Can you work these out from the model? Positions are in its coordinate system, mm. Face numbers are marked on the shaded views. Give positions to 0.01 mm unless a question says otherwise; leave off trailing zeros. Write each loop counter-clockwise with the first axis right and the second up, starting at its lowest first coordinate (ties: lowest second). Pieces come first, ordered by that corner, then holes.
Autodesk Inventor part; units mm, degrees
ref_plane "YZ Plane" through (0, 0, 0) normal (1, 0, 0) x (0, 1, 0)
ref_plane "XZ Plane" through (0, 0, 0) normal (0, 1, 0) x (-1, 0, 0)
ref_plane "XY Plane" through (0, 0, 0) normal (0, 0, 1) x (1, 0, 0)
sketch "Sketch1" plane through (-26.51, 3.1066, 0) normal (0, 0, 1) x (1, 0, 0)
  circle A0 centre (0, 0) radius 7.62 construction
  circle A1 centre (0, 0) radius 9.75
  circle A2 centre (33.02, 0) radius 25.4 construction
  line L0 (0, 0) -> (7.62, 0)
  line L1 (0, 0) -> (7.62, 0) construction
  circle A3 centre (33.02, 0) radius 9.5
  line L2 (0, -30) -> (33.02, -30)
  line L3 (33.02, 30) -> (0, 30)
  arc A4 (33.02, -30) -> (63.02, 0) centre (33.02, 0) ccw
  arc A5 (0, 30) -> (0, -30) centre (0, 0) ccw
  circle A6 centre (0, 0) radius 25.4 construction
  line L4 (0, 25.4) -> (0, 0) construction
  line L5 (0, 25.4) -> (25.4, 25.4) construction
  circle A7 centre (0, 25.4) radius 2.2
  circle A8 centre (-21.997, 12.7) radius 2.2
  circle A9 centre (-21.997, -12.7) radius 2.2
  circle A10 centre (0, -25.4) radius 2.2
  circle A11 centre (21.997, -12.7) radius 2.2
  circle A12 centre (21.997, 12.7) radius 2.2
  line L6 (63.02, 0) -> (63.02, 30)
  line L7 (63.02, 30) -> (33.02, 30)
  circle A13 centre (58.02, 25) radius 2.2
  circle A14 centre (73.02, 0) radius 2.75
  circle A15 centre (73.02, 0) radius 10
  line L8 (81.02, 6) -> (63.02, 30)
  line L9 (78.02, -8.6603) -> (48.02, -25.9808)
  dimension "d13" = 50.8
  dimension "d21" = 15.24
  dimension "d20" = 19.5
  dimension "d18" = 50.8
  dimension "d17" = 7.62
  dimension "d25" = 0
  dimension "d19" = 33.02
  dimension "d16" = 19
  dimension "d14" = 30
  dimension "d15" = 60
  dimension "d26" = 25.4
  dimension "d27" = 90
  dimension "d12" = 4.4
  dimension "d2" = 360
  dimension "d11" = 30
  dimension "d9" = 30
  dimension "d10" = 90
  dimension "d6" = 4.4
  dimension "d8" = 5
  dimension "d7" = 5
  dimension "d4" = 5.5
  dimension "d5" = 10
  dimension "d3" = 20
extrude "Extrusion1" add sketch "Sketch1" along normal blind 7 contours A5 L3 L7 L6 A4 L2 | A4 A15 L9 | L6 L8 A15 | A15 | A11 | A12
fillet "Fillet1" radius 10 1 edges at (36.51, 33.1066, 3.5)
sketch "Sketch2" plane through (-26.51, 3.1066, 7) normal (0, 0, 1) x (1, 0, 0)
  circle A0 centre (0, 25.4) radius 2.2
  circle A1 centre (0, -25.4) radius 2.2
  circle A2 centre (58.02, 25) radius 2.2
  point P0 (26.51, -3.1066)
hole "Hole1" at (-26.51, 28.5066, 7) at (31.51, 28.1066, 7) at (-26.51, -22.2934, 7) direction (0, 0, -1) diameter 4.4 depth 7 countersink diameter 8.13 countersink angle 82
properties part number "Outer Plate" material "Aluminum 6061"
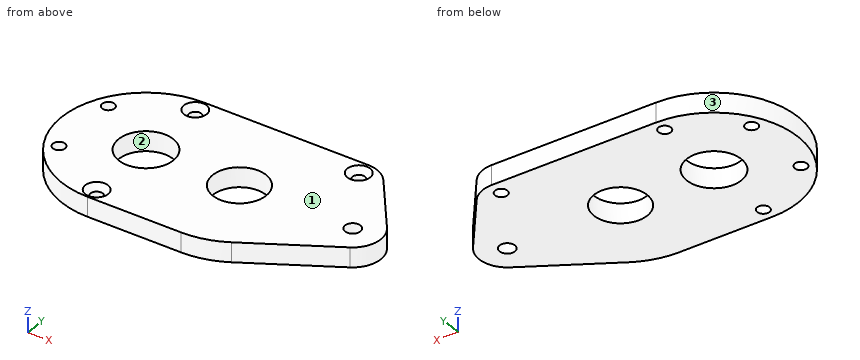
1) Suppose I cut it at D-D on x = 18. Write out the boundary of the cut face in (y, z), plus the area to 3 significant figures.
Values follow:
outline: (-24.61, 0) - (33.11, 0) - (33.11, 7) - (-24.61, 7) - close
area: 404 mm2
2) If we mould it in two halves opening along X, with no side actions, what happens to the marked faces 1, 2 and 3? For each: +X half, -X half, draft (parallel to the pull), parting line (faces both ways), or undercut.
Values follow:
face 1: draft
face 2: undercut
face 3: -X half
3) Suppose I cut it at C-C on x = 46.51. Write out the boundary of the cut face in (y, z), plus the area to 3 significant figures.
Values follow:
outline: (-8.44, 0) - (0.36, 0) - (0.36, 7) - (-8.44, 7) - close; (5.86, 0) - (19.77, 0) - (19.77, 7) - (5.86, 7) - close
area: 159 mm2
4) For pin 1 Ø3 at (y, z) = (7, 3) entering from +X; pin 2 Ø2 at (x, y) = (23.5, -18) entering from -Z; pin 3 Ø3 at (x, z) = (-42.5, 4) entering from +Y, each with a flat end and sliding along its axis, tell me the tip position at first contact or that it passes through.
Values follow:
pin 1: stops at x = 56.22
pin 2: stops at z = 0
pin 3: stops at y = 29.38
5) Suppose I cut it at B-B on z = 1.25. State how many separate pieces and enclosed holes the cut face has, plus the area to 3 significant figures.
Values follow:
separate pieces: 1
enclosed holes: 8
area: 4,920 mm2
6) Suppose I cut it at A-A on y = -2.5. Write out the boundary of the cut face in (x, z).
Values follow:
outline: (-55.98, 0) - (-34.49, 0) - (-34.49, 7) - (-55.98, 7) - close; (-18.53, 0) - (-1.16, 0) - (-1.16, 7) - (-18.53, 7) - close; (14.18, 0) - (54.79, 0) - (54.79, 7) - (14.18, 7) - close
7) Please list where these lines run through material, in increasing order: L1, parallel to Y at x = -26.51, z = 3.25; L2, parallel to X at y = 8.5, z = 3.5; L3, parallel to Y at x = -46.5, z = 6.75.
Values follow:
L1: y = -26.89 to -24.49, -20.09 to -6.64, 12.86 to 26.31, 30.71 to 33.11
L2: x = -56.02 to -34.63, -18.39 to -1.31, 14.33 to 54.93
L3: y = -19.26 to -10.49, -8.69 to 14.91, 16.71 to 25.48
